from build123d import *

# Parameters (mm, degrees)
F2_R     = 2.5
F2_R_2   = 15.5
F3_DEPTH = 12
F5_DEPTH = 7.1


with BuildPart() as f3:
    # F2 (on offset) → F3 (new body)
    with BuildSketch(Plane.XY.offset(-19)):
        with BuildLine():
            ThreePointArc((-22, 2), (-23.464466, -1.535534), (-27, -3))
            Line((-27, -3), (-66.61081, -3))
            ThreePointArc((-66.61081, -3), (0, -54), (66.61081, -3))
            Line((66.61081, -3), (27, -3))
            ThreePointArc((27, -3), (23.464466, -1.535534), (22, 2))
            Line((22, 2), (22, 30.368569))
            ThreePointArc((22, 30.368569), (0, 37.5), (-22, 30.368569))
            Line((-22, 30.368569), (-22, 2))
        make_face()
        with Locations((-15, -25)):
            Circle(F2_R, mode=Mode.SUBTRACT)
        with Locations((0, -30)):
            Circle(F2_R, mode=Mode.SUBTRACT)
        with Locations((15, -25)):
            Circle(F2_R, mode=Mode.SUBTRACT)
        with Locations((-15, 25)):
            Circle(F2_R, mode=Mode.SUBTRACT)
        Circle(F2_R_2, mode=Mode.SUBTRACT)
        with Locations((15, 25)):
            Circle(F2_R, mode=Mode.SUBTRACT)
        with Locations((0, 30)):
            Circle(F2_R, mode=Mode.SUBTRACT)
    extrude(amount=-F3_DEPTH)

    # F4 (on offset) → F5 (cut)
    with BuildSketch(Plane.XY.offset(-19)):
        with BuildLine():
            ThreePointArc((3, 20), (0, 23), (-3, 20))
            Line((-3, 20), (-3, 0))
            Line((-3, 0), (-3, -20))
            ThreePointArc((-3, -20), (0, -23), (3, -20))
            Line((3, -20), (3, 0))
            Line((3, 0), (3, 20))
        make_face()
    extrude(amount=-F5_DEPTH, mode=Mode.SUBTRACT)


solid = f3.part
Geometry check sheet. Reference: the model listing, model coordinates, mm. A direction names the side the tool comes from. Coordinates: 2 decimals unless noted, no trailing zeros. Order: outer loops, then holes, each group sorted by start corner. A loop starts at its lowest first (then second) coordinate and runs counter-clockwise, first axis right, second up. Notation, with made-up numbers: (86, 56) -> (106, 56) arc R20 ccw to (106, 91) -> close; hole circle Ø7 at (13.5, 82.5). An arc over 180 degrees is marked (long way). Use a Markdown table: item, result. Add a question column.
1. Cross-section at C-C (y = -12). Enter the section's corners in (x, z).
2. Cross-section at B-B (y = 0). Enter the section's corners in (x, z), and give its area (3 significant figures).
3. Set-up check for faces 4 (the face through (-1.26, -53.99, -24.92)), 5 (the face through (47, -3, -25)), 6 (the face through (0, -23, -23)): record each of +Z, -Z, +X, -X, +Y, -Y from which the full face is reachable in a straight line by a thin tool's end or side.
4. Go/stop test with flat-tipped pins: pin 1 Ø3 at (x, y) = (0, 30) entering from -Z; pin 2 Ø5 at (x, z) = (-30.5, -21.5) entering from +Y; pin 3 Ø2 at (y, z) = (4, -23.5) entering from +X; pin 4 Ø1.5 at (y, z) = (-39.5, -21) entering from -X. Record where each tip stops, or that it passes through.
5. Cross-section at A-A (z = -27.75). Enter the section's corners in (x, y).
6. Material ranges on L1, parallel to Y at x = 0, z = -22; L2, parallel to X at y = -24, z = -23.75; L3, parallel to Y at x = 12, z = -20.5, recorded low to high.
7. Mould release check, pull along X, two halves, no side actions. Record for faces 1 (the face through (-3, -18, -23)), 2 (the face through (24, -2, -25)), 3 (the face through (-47, -3, -25)): pulls with the +X half, pulls with the -X half, needs draft (parallel to the pull), parting line crosses it, or undercut.
8. Cross-section at D-D (x = -52). Enter the section's corners in (y, z), and give its area (3 significant figures).
Filled sheet:
| question | item | result |
|---|---|---|
| 1 | outline | (-63.5, -31) -> (-9.81, -31) -> (-9.81, -19) -> (-63.5, -19) -> close; (9.81, -31) -> (63.5, -31) -> (63.5, -19) -> (9.81, -19) -> close |
| 2 | outline | (-22.42, -31) -> (-15.5, -31) -> (-15.5, -19) -> (-22.42, -19) -> close; (15.5, -31) -> (22.42, -31) -> (22.42, -19) -> (15.5, -19) -> close |
| 2 | area | 166 mm2 |
| 3 | face 4 | +Z, -Z, -Y |
| 3 | face 5 | +Z, -Z, +X, +Y |
| 3 | face 6 | +Z |
| 4 | pin 1 | through |
| 4 | pin 2 | y = -3 |
| 4 | pin 3 | x = 22 |
| 4 | pin 4 | x = -43.27 |
| 5 | outline | (-66.61, -3) arc R69 ccw to (66.61, -3) -> (27, -3) arc R5 cw to (22, 2) -> (22, 30.37) arc R37.5 ccw to (-22, 30.37) -> (-22, 2) arc R5 cw to (-27, -3) -> close; hole circle Ø5 at (-15, -25); hole circle Ø5 at (-15, 25); hole circle Ø31 at (0, 0); hole circle Ø5 at (0, -30); hole circle Ø5 at (0, 30); hole circle Ø5 at (15, -25); hole circle Ø5 at (15, 25) |
| 6 | L1 | -54 to -32.5, -27.5 to -23, 23 to 27.5, 32.5 to 37.5 |
| 6 | L2 | -56.92 to -17.29, -12.71 to 12.71, 17.29 to 56.92 |
| 6 | L3 | -52.95 to -9.81, 9.81 to 35.53 |
| 7 | face 1 | undercut |
| 7 | face 2 | pulls with the +X half |
| 7 | face 3 | needs draft |
| 8 | outline | (-30.35, -31) -> (-3, -31) -> (-3, -19) -> (-30.35, -19) -> close |
| 8 | area | 328 mm2 |
